```python
from build123d import *

# Parameters (mm, degrees)
F1_DEPTH = 10
F3_DEPTH = 10


with BuildPart() as f1:
    # F0 (on Top) → F1 (new body)
    with BuildSketch(Plane.XY):
        with BuildLine():
            ThreePointArc((-7.2758161054, -8.25), (-8.5128273031, -6.966474812), (-9.5262794416, -5.5))
            Line((-9.5262794416, -5.5), (-20, -5.5))
            Line((-20, -5.5), (-20, -8.25))
            Line((-20, -8.25), (-7.2758161054, -8.25))
        make_face()
        with BuildLine():
            ThreePointArc((0, -11), (-3.8890872965, -10.2895578136), (-7.2758161054, -8.25))
            Line((-7.2758161054, -8.25), (-20, -8.25))
            Line((-20, -8.25), (-20, -11))
            Line((-20, -11), (0, -11))
        make_face()
        with BuildLine():
            Line((0, -5.5), (-9.5262794416, -5.5))
            ThreePointArc((-9.5262794416, -5.5), (-8.5128273031, -6.966474812), (-7.2758161054, -8.25))
            Line((-7.2758161054, -8.25), (-1.625, -8.25))
            ThreePointArc((-1.625, -8.25), (-1.1490485194, -7.1009514806), (0, -6.625))
            Line((0, -6.625), (0, -5.5))
        make_face()
        with BuildLine():
            Line((-1.625, -8.25), (-7.2758161054, -8.25))
            ThreePointArc((-7.2758161054, -8.25), (-3.8890872965, -10.2895578136), (0, -11))
            Line((0, -11), (0, -9.875))
            ThreePointArc((0, -9.875), (-1.1490485194, -9.3990485194), (-1.625, -8.25))
        make_face()
        with BuildLine():
            ThreePointArc((0, -11), (3.8890872965, -10.2895578136), (7.2758161054, -8.25))
            Line((7.2758161054, -8.25), (1.625, -8.25))
            ThreePointArc((1.625, -8.25), (1.1490485194, -9.3990485194), (0, -9.875))
            Line((0, -9.875), (0, -11))
        make_face()
        with BuildLine():
            ThreePointArc((7.2758161054, -8.25), (8.5128273031, -6.966474812), (9.5262794416, -5.5))
            Line((9.5262794416, -5.5), (0, -5.5))
            Line((0, -5.5), (0, -6.625))
            ThreePointArc((0, -6.625), (1.1490485194, -7.1009514806), (1.625, -8.25))
            Line((1.625, -8.25), (7.2758161054, -8.25))
        make_face()
        with BuildLine():
            Line((20, -5.5), (9.5262794416, -5.5))
            ThreePointArc((9.5262794416, -5.5), (8.5128273031, -6.966474812), (7.2758161054, -8.25))
            Line((7.2758161054, -8.25), (20, -8.25))
            Line((20, -8.25), (20, -5.5))
        make_face()
        with BuildLine():
            Line((20, -8.25), (7.2758161054, -8.25))
            ThreePointArc((7.2758161054, -8.25), (3.8890872965, -10.2895578136), (0, -11))
            Line((0, -11), (20, -11))
            Line((20, -11), (20, -8.25))
        make_face()
        with BuildLine():
            ThreePointArc((9.5262794416, -5.5), (10.6251840892, -2.8470094961), (11, 0))
            Line((11, 0), (5.25, 0))
            ThreePointArc((5.25, 0), (-3.7123106012, -3.7123106012), (0, 5.25))
            Line((0, 5.25), (0, 5.5))
            Line((0, 5.5), (0, 6.625))
            ThreePointArc((0, 6.625), (-1.625, 8.25), (0, 9.875))
            Line((0, 9.875), (0, 11))
            ThreePointArc((0, 11), (-9.5262794416, 5.5), (-9.5262794416, -5.5))
            Line((-9.5262794416, -5.5), (0, -5.5))
            Line((0, -5.5), (9.5262794416, -5.5))
        make_face()
        with BuildLine():
            Line((5.25, 0), (11, 0))
            ThreePointArc((11, 0), (7.7781745931, 7.7781745931), (0, 11))
            Line((0, 11), (0, 9.875))
            ThreePointArc((0, 9.875), (1.1490485194, 9.3990485194), (1.625, 8.25))
            ThreePointArc((1.625, 8.25), (1.1490485194, 7.1009514806), (0, 6.625))
            Line((0, 6.625), (0, 5.5))
            Line((0, 5.5), (0, 5.25))
            ThreePointArc((0, 5.25), (3.7123106012, 3.7123106012), (5.25, 0))
        make_face()
        Polygon((20, -11), (0, -11), (-20, -11), (-20, -14), (20, -14), align=None)
    extrude(amount=F1_DEPTH)

    # F2 (on face) → F3 (cut)
    with BuildSketch(Plane.XZ.offset(14)):
        with BuildLine():
            Line((-17, 5), (-13, 5))
            ThreePointArc((-13, 5), (-15, 7), (-17, 5))
        make_face()
        with BuildLine():
            ThreePointArc((-17, 5), (-15, 3), (-13, 5))
            Line((-13, 5), (-17, 5))
        make_face()
        with BuildLine():
            Line((13, 5), (17, 5))
            ThreePointArc((17, 5), (15, 7), (13, 5))
        make_face()
        with BuildLine():
            ThreePointArc((13, 5), (15, 3), (17, 5))
            Line((17, 5), (13, 5))
        make_face()
    extrude(amount=-F3_DEPTH, mode=Mode.SUBTRACT)


solid = f1.part
```
Could you check a few things on this model? Use its own coordinates, in mm. A direction names the side the tool comes from. Round coordinates to 2 decimals unless told otherwise and drop trailing zeros. Write each loop counter-clockwise with the first axis right and the second up, starting at its lowest first coordinate (ties: lowest second). Pieces come first, ordered by that corner, then holes.
(1) Suppose I cut it at D-D on y = 9. Write out the boundary of the cut face in (x, z), and give its area (3 significant figures).
Findings below:
outline: (-6.32, 0) - (-1.44, 0) - (-1.44, 10) - (-6.32, 10) - close; (1.44, 0) - (6.32, 0) - (6.32, 10) - (1.44, 10) - close
area: 97.7 mm2
(2) For pin 1 (5 mm diameter, centred on x = 15.5, z = 6.5, fed in from +Y); pin 2 (1 mm diameter, centred on x = -9, z = 3, fed in from +Y); pin 3 (3 mm diameter, centred on x = -6, z = 5, fed in from +Y), each with a flat end and sliding along its axis, tell me the tip position at first contact or that it passes through.
Findings below:
pin 1: stops at y = -5.5
pin 2: stops at y = 6.98
pin 3: stops at y = 10.04
(3) Suppose I cut it at B-B on x = -15. Write out the boundary of the cut face in (y, z).
Findings below:
outline: (-14, 0) - (-5.5, 0) - (-5.5, 3) - (-14, 3) - close; (-14, 7) - (-5.5, 7) - (-5.5, 10) - (-14, 10) - close
(4) Suppose I cut it at A-A on z = 5. Write out the boundary of the cut face in (x, y) (3 decimals).
Findings below:
outline: (-20, -14) - (-17, -14) - (-17, -5.5) - (-20, -5.5) - close; (-13, -14) - (13, -14) - (13, -5.5) - (9.526, -5.5) arc R11 ccw (long way) to (-9.526, -5.5) - (-13, -5.5) - close; (17, -14) - (20, -14) - (20, -5.5) - (17, -5.5) - close; hole circle Ø10.5 at (0, 0); hole circle Ø3.25 at (0, -8.25); hole circle Ø3.25 at (0, 8.25)
(5) Thinking about a two-plate mould opening in X: for faces 1 (the face through (14.8, -5.5, 2.7)), 2 (the face through (-20, -10, 5)), 3 (the face through (16.6, -9.8, 6.2)), which applies, +X half, -X half, draft (parallel to the pull), parting line (faces both ways), or undercut?
Findings below:
face 1: draft
face 2: -X half
face 3: undercut
(6) Which directions (+Z, -Z, +X, -X, +Y, -Y) give clear straight access to the entire face, cutting with the end or side of a thin tool? Please do faces 4 (the face through (20, -10, 5)), 5 (the face through (-14.7, -5.5, 2.7)).
Findings below:
face 4: +Z, -Z, +X, +Y, -Y
face 5: +Z, -Z, -X
(7) Suppose I cut it at C-C on z = 8. Write out the boundary of the cut face in (x, y) (3 decimals).
Findings below:
outline: (-20, -14) - (20, -14) - (20, -5.5) - (9.526, -5.5) arc R11 ccw (long way) to (-9.526, -5.5) - (-20, -5.5) - close; hole circle Ø10.5 at (0, 0); hole circle Ø3.25 at (0, -8.25); hole circle Ø3.25 at (0, 8.25)
(8) If I drill on probe 1 along X at (y, z) = (-10.5, 5); probe 2 along X at (y, z) = (0, 6.5); probe 3 along Z at (x, y) = (15, -8), over which ranges is the centre line in solid material (lowest first)?
Findings below:
probe 1: x = -20 to -17, -13 to 13, 17 to 20
probe 2: x = -11 to -5.25, 5.25 to 11
probe 3: z = 0 to 3, 7 to 10
